```python
from build123d import *

# Parameters (mm, degrees)
EXTRUDE_1_DEPTH     = 70
SKETCH_3_R          = 10
CUT_EXTRUDE_1_DEPTH = 70


with BuildPart() as part:
    # 스케치1 → 보스-돌출1 (new body)
    with BuildSketch(Plane(origin=(0, 0, 0), x_dir=(0, 0, -1), z_dir=(1, 0, 0))):
        Polygon((0, 0), (40, 0), (40, 40), (20, 40), (20, 20), (0, 20), align=None)
    extrude(amount=-EXTRUDE_1_DEPTH)

    # 스케치3 → 컷-돌출1 (cut)
    with BuildSketch(Plane(origin=(0, 0, -40), x_dir=(-1, 0, 0), z_dir=(0, 0, -1))):
        with Locations((50, 20)):
            Circle(SKETCH_3_R)
        Polygon((0, 0), (40, 40), (0, 40), align=None)
    extrude(amount=-CUT_EXTRUDE_1_DEPTH, mode=Mode.SUBTRACT)


solid = part.part
```
Read the model definition and answer for the solid it produces. Units are mm, in the model's axes. A direction names the side the tool comes from. Coordinates: 2 decimals unless noted, no trailing zeros. Write each loop counter-clockwise with the first axis right and the second up, starting at its lowest first coordinate (ties: lowest second). Pieces come first, ordered by that corner, then holes. Notation, with made-up numbers: (5.25, 23.5) -> (13.25, 23.5) arc R15 cw to (13.25, 27.5) -> close; hole circle Ø11 at (66, 49). An arc over 180 degrees is marked (long way). Return JSON: item names as keys, results as strings.
1. A cutting plane is placed at C-C (y = 22.5). Determine the outline of the cut face in (x, z), and give its area (3 significant figures).
Found:
{"outline": "(-70, -40) -> (-59.68, -40) -> (-59.68, -20) -> (-70, -20) -> close; (-40.32, -40) -> (-22.5, -40) -> (-22.5, -20) -> (-40.32, -20) -> close", "area": "563 mm2"}
2. Find the intervals of material crossed by line 1 along X through (y, z) = (20, -24); line 2 along Y through (x, z) = (-50, -31); line 3 along Y through (x, z) = (-54, -35), in increasing order. Write a range as from..to.
Found:
{"line 1": "-70..-60, -40..-20", "line 2": "0..10, 30..40", "line 3": "0..10.83, 29.17..40"}
3. A cutting plane is placed at D-D (x = -31.5). Determine the outline of the cut face in (y, z).
Found:
{"outline": "(0, -40) -> (31.5, -40) -> (31.5, -20) -> (20, -20) -> (20, 0) -> (0, 0) -> close"}
4. A tool of negligible diameter and unlimited length cuts with its end or side. For faces 1 (the face through (-55, 40, -30)), 2 (the face through (-65, 20, -10)), from which of +Z, -Z, +X, -X, +Y, -Y can it reach the whole face along a straight path? Write none if from no direction.
Found:
{"face 1": "+Z, -Z, +X, -X, +Y", "face 2": "+Z, +X, -X, +Y"}
5. Determine the mould class of faces 3 (the face through (-47.83, 10.24, -24.72)), 4 (the face through (-15, 15, -25)), 5 (the face through (-70, 16, -24)), 6 (the face through (-50, 32, -20)) for opening direction X: pulls with the +X half, pulls with the -X half, needs draft (parallel to the pull), parting line crosses it, or undercut.
Found:
{"face 3": "undercut", "face 4": "pulls with the +X half", "face 5": "pulls with the -X half", "face 6": "needs draft"}
6. Each of these flat-tipped pins is pushed along its axis until it touches: P1, Ø11, axis at x = -64, z = -7, coming from the +Y side; P2, Ø5, axis at x = -28.5, y = 33.5, coming from the -Z side; P3, Ø22, axis at x = -52, y = 28.5, coming from the +Z side; P4, Ø3, axis at x = -20, z = -19, coming from the +Y side. Where does it stop, or does it pass through?
Found:
{"P1": "y = 20", "P2": "through", "P3": "z = -20", "P4": "y = 21.12"}
7. A cutting plane is placed at B-B (z = -33). Determine the outline of the cut face in (x, y).
Found:
{"outline": "(-70, 0) -> (0, 0) -> (-40, 40) -> (-70, 40) -> close; hole circle Ø20 at (-50, 20)"}
8. A cutting plane is placed at A-A (x = -50). Determine the outline of the cut face in (y, z), and give its area (3 significant figures).
Found:
{"outline": "(0, -40) -> (10, -40) -> (10, 0) -> (0, 0) -> close; (30, -40) -> (40, -40) -> (40, -20) -> (30, -20) -> close", "area": "600 mm2"}
